Build history of the part. All positions in model axes, mm. Face numbers are marked on the shaded views. Round coordinates to 2 decimals unless told otherwise and drop trailing zeros. Order: outer loops, then holes, each group sorted by start corner. A loop starts at its lowest first (then second) coordinate and runs counter-clockwise, first axis right, second up. Notation, with made-up numbers: M 9.5,29.5 L 42.5,29.5 A12 ccw 42.5,45.5 Z; hole C 48,-39.75 d8. An arc over 180 degrees is marked long. One line per item, written item: value. Start each with the question number.
Item 1: Probe L1, parallel to X at y = 21, z = 3.1; L2, parallel to Y at x = -4.75, z = 2.75; L3, parallel to X at y = 50.5, z = 3.1. List the from-to ranges inside material, lowest first.
Item 2: Pin check, flat tips, straight feed: pin 1 (1.2 mm diameter, centred on y = 66, z = 3, fed in from -X); pin 2 (4 mm diameter, centred on x = -4.75, y = 21, fed in from -Z); pin 3 (1.5 mm diameter, centred on x = -24.5, z = 3.5, fed in from +Y). Stop position of each tip, or through.
Item 3: Band-saw the part on C-C, the plane x = -36.75. Write the cut outline in (y, z) (3 decimals), then the cut area to 3 significant figures.
Item 4: Band-saw the part on A-A, the plane y = 82.5. Write the cut outline in (x, z) (3 decimals), then the cut area to 3 significant figures.
Item 5: Band-saw the part on D-D, the plane y = 35.5. Write the cut outline in (x, z).
Item 6: Band-saw the part on B-B, the plane z = 1.15. Give the number of separate pieces and of enclosed holes in the cut face, then the cut area to 3 significant figures.
Item 7: Two-plate mould, pull along Z, no slides. Class the marked faces 1 and 2: +Z half, -Z half, draft (parallel to the pull), parting line (faces both ways), or undercut.
```python
from build123d import *

# Parameters (mm, degrees)
EXTRUDE_1_DEPTH                = 4
HOLE_WIZARD_M2_5_1_D           = 2.9
HOLE_WIZARD_M2_5_1_CSINK_D     = 2.95
HOLE_WIZARD_M2_5_1_CSINK_ANGLE = 90
FILLET_2_R                     = 3


with BuildPart() as part:
    # 草图1 → 凸台-拉伸1 (new body)
    with BuildSketch(Plane.XY):
        Polygon((0, 0), (-41.5, 0), (-41.5, 25.5), (-13.75, 48.5), (-13.75, 90), (16.25, 90), (16.25, 0), align=None)
    extrude(amount=EXTRUDE_1_DEPTH)

    # M2.5 间隙孔1 (through all)
    with Locations(Plane.XY.offset(4)):
        with Locations((9.25, 50.5), (-36.75, 5), (-36.75, 21), (-4.75, 5), (-4.75, 21), (-6.75, 82.5), (9.25, 82.5), (-6.75, 50.5)):
            CounterSinkHole(HOLE_WIZARD_M2_5_1_D / 2, HOLE_WIZARD_M2_5_1_CSINK_D / 2, counter_sink_angle=HOLE_WIZARD_M2_5_1_CSINK_ANGLE)

    # 圆角2
    fillet_2_edges = [part.edges().sort_by_distance(p)[0] for p in [
        (-41.5, 0, 2),
        (-41.5, 25.5, 2),
        (-13.75, 48.5, 2),
        (-13.75, 90, 2),
        (16.25, 90, 2),
        (16.25, 0, 2),
    ]]
    fillet(fillet_2_edges, radius=FILLET_2_R)


solid = part.part
```
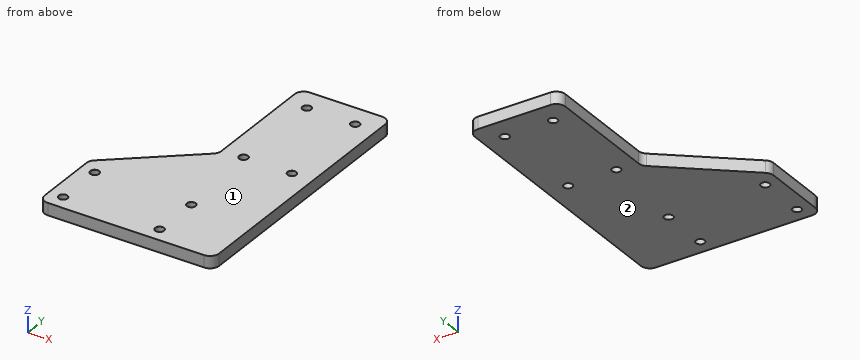
Output:
1. L1: x = -41.5 to -38.2, -35.3 to -6.2, -3.3 to 16.25
1. L2: y = 0 to 3.55, 6.45 to 19.55, 22.45 to 90
1. L3: x = -13.75 to -8.2, -5.3 to 7.8, 10.7 to 16.25
2. pin 1: stops at x = -13.75
2. pin 2: stops at z = 0
2. pin 3: stops at y = 40.21
3. outline: M 0,0 L 3.55,0 L 3.55,3.975 L 3.525,4 L 0,4 Z; M 6.45,0 L 19.55,0 L 19.55,3.975 L 19.525,4 L 6.475,4 L 6.45,3.975 Z; M 22.45,0 L 29.437,0 L 29.437,4 L 22.475,4 L 22.45,3.975 Z
3. area: 94.5 mm²
4. outline: M -13.75,0 L -8.2,0 L -8.2,3.975 L -8.225,4 L -13.75,4 Z; M -5.3,0 L 7.8,0 L 7.8,3.975 L 7.775,4 L -5.275,4 L -5.3,3.975 Z; M 10.7,0 L 16.25,0 L 16.25,4 L 10.725,4 L 10.7,3.975 Z
4. area: 96.8 mm²
5. outline: M -29.43,0 L 16.25,0 L 16.25,4 L -29.43,4 Z
6. separate pieces: 1
6. enclosed holes: 8
6. area: 3,670 mm²
7. face 1: +Z half
7. face 2: -Z half
